```python
from build123d import *

# Parameters (mm, degrees)
ESQUISSE2_R             = 1
ESQUISSE2_R_2           = 3
ENL_V_MAT_EXTRU_1_DEPTH = 21.184253764
ESQUISSE4_R             = 1
ENL_V_MAT_EXTRU_2_DEPTH = 21.184253764


with BuildPart() as part:
    # Esquisse1 → Révolution1 (revolve)
    with BuildSketch(Plane.XY):
        Polygon((0, 0), (0, 12.7), (5.08, 12.7), (5.08, 6.035), (9.21, 6.035), (9.21, 0), align=None)
    revolve(axis=Axis((9.21, 0, 0), (-1, 0, 0)))

    # Esquisse2 → Enlèv. mat.-Extru.1 (cut, through all)
    with BuildSketch(Plane.ZY):
        with Locations(Location((9.53, 0, 0), (0, 0, 270))):
            Circle(ESQUISSE2_R)
        with Locations(Location((4.765, -8.253222098, 0), (0, 0, 270))):
            Circle(ESQUISSE2_R)
        with Locations(Location((-4.765, -8.253222098, 0), (0, 0, 270))):
            Circle(ESQUISSE2_R)
        with Locations(Location((-9.53, 0, 0), (0, 0, 270))):
            Circle(ESQUISSE2_R)
        with Locations(Location((-4.765, 8.253222098, 0), (0, 0, 270))):
            Circle(ESQUISSE2_R)
        with Locations(Location((4.765, 8.253222098, 0), (0, 0, 270))):
            Circle(ESQUISSE2_R)
        with Locations(Location((0, 0, 0), (0, 0, 270))):
            Circle(ESQUISSE2_R_2)
    extrude(amount=-ENL_V_MAT_EXTRU_1_DEPTH, mode=Mode.SUBTRACT)

    # Esquisse4 → Enlèv. mat.-Extru.2 (cut, through all)
    with BuildSketch(Plane(origin=(0, 0, 0), x_dir=(1, 0, 0), z_dir=(0, 1, 0))):
        with Locations(Location((2.54, 0, 0), (0, 0, 90))):
            Circle(ESQUISSE4_R)
        with Locations(Location((7.145, 0, 0), (0, 0, 90))):
            Circle(ESQUISSE4_R)
    extrude(amount=ENL_V_MAT_EXTRU_2_DEPTH, mode=Mode.SUBTRACT)


solid = part.part
```
Check sheet for the modelled part. Datum: model origin and axes. Units: mm. A direction names the side the tool comes from. Coordinates: 2 decimals unless noted, no trailing zeros. Loops run counter-clockwise (first coordinate to the right, second up) from the corner with the lowest first, then second, coordinate; pieces in that order, holes last. Notation, with made-up numbers: M 58,-6.75 L 98,-6.75 A35 cw 98,28.25 Z; hole C 29.5,55 d11. An arc over 180 degrees is marked long. Answer as a JSON object with one key per item and string values.
1. Depth check by flat-ended pin: P1, Ø2.5, axis at y = 0, z = -9.53, coming from the -X side; P2, Ø1, axis at x = 3.5, z = -3, coming from the +Y side; P3, Ø1, axis at x = 3.5, y = -6.5, coming from the +Z side; P4, Ø2.5, axis at y = 8.25, z = -4.76, coming from the +X side. Enter the tip coordinate at first touch or a pass-through.
Outcome:
{"P1": "x = 0", "P2": "y = 12.45", "P3": "z = 11.19", "P4": "x = 5.08"}
2. Sectioned sample at B-B on y = 0. Record the cut outline in (x, z) (3 decimals).
Outcome:
{"outline": "M 0,-12.7 L 5.08,-12.7 L 5.08,-10.53 L 0,-10.53 Z; M 0,-8.53 L 5.08,-8.53 L 5.08,-6.035 L 9.21,-6.035 L 9.21,-3 L 0,-3 Z; M 0,3 L 9.21,3 L 9.21,6.035 L 5.08,6.035 L 5.08,8.53 L 0,8.53 Z; M 0,10.53 L 5.08,10.53 L 5.08,12.7 L 0,12.7 Z"}
3. Release check for a two-part mould opening along Z. For faces 3 (the cylindrical face through (2.504, -8.715, 3.878)), 4 (the flat face through (5.08, 5.5, -3)), 5 (the cylindrical face through (7.17, -1.31, 5.89)) record: pulls with the +Z half, pulls with the -Z half, needs draft (parallel to the pull), parting line crosses it, or undercut.
Outcome:
{"face 3": "undercut", "face 4": "needs draft", "face 5": "parting line crosses it"}
4. Sectioned sample at C-C on z = 9.53. Record the cut outline in (x, y).
Outcome:
{"outline": "M 0,-8.39 L 5.08,-8.39 L 5.08,-1 L 0,-1 Z; M 0,1 L 5.08,1 L 5.08,8.39 L 0,8.39 Z"}
5. Scan lines: L1, parallel to X at y = 3.7, z = 0 (3 decimals); L2, parallel to Y at x = 4, z = -5.25; L3, parallel to X at y = -2.25, z = -6.5. Record each from-to range of solid material in increasing order. Write a range as from..to.
Outcome:
{"L1": "0..1.54, 3.54..6.145, 8.145..9.21", "L2": "-11.56..-9.13, -7.38..7.38, 9.13..11.56", "L3": "0..5.08"}
6. Access from +Z, -Z, +X, -X, +Y, -Y to the whole of each face (thin tool, end or side, straight path). Record for faces 1 (the cylindrical face through (2.504, 0.217, 8.554)), 2 (the cylindrical face through (6.845, 4.409, -0.954)).
Outcome:
{"face 1": "+X, -X", "face 2": "+Y"}
7. Sectioned sample at D-D on x = 5.5. Record the cut outline in (y, z) (3 decimals).
Outcome:
{"outline": "C 0,0 d12.07; hole C 0,0 d6"}
8. Sectioned sample at A-A on z = 0. Record the cut outline in (x, y) (3 decimals).
Outcome:
{"outline": "M 0,-12.7 L 5.08,-12.7 L 5.08,-6.035 L 9.21,-6.035 L 9.21,-3 L 0,-3 Z; M 0,3 L 1.54,3 L 1.54,12.7 L 0,12.7 Z; M 3.54,3 L 6.145,3 L 6.145,6.035 L 5.08,6.035 L 5.08,12.7 L 3.54,12.7 Z; M 8.145,3 L 9.21,3 L 9.21,6.035 L 8.145,6.035 Z"}
